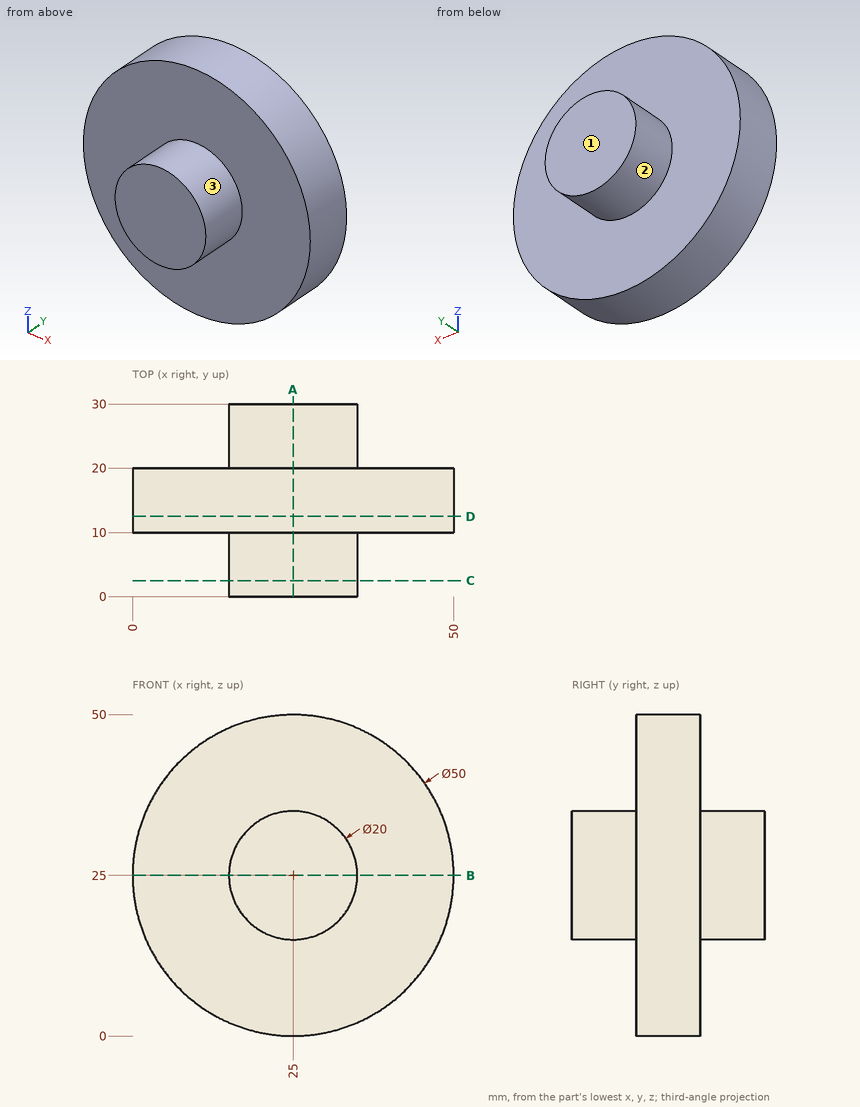
Can you work these out from the drawing? Everything is in mm from the part's minimum corner. A direction names the side the tool comes from. Round coordinates to 2 decimals unless told otherwise and drop trailing zeros. Loops run counter-clockwise (first coordinate to the right, second up) from the corner with the lowest first, then second, coordinate; pieces in that order, holes last. Notation, with made-up numbers: (63.5, 19.25) -> (110.5, 19.25) arc R23 cw to (110.5, 38.25) -> close; hole circle Ø9 at (-6.5, 45). An arc over 180 degrees is marked (long way). Use CSV: the item, a comma, the result in double quotes.
(1) Will these pins go through, and if not, where does the flat tip stop? pin 1 Ø10 at (x, y) = (26, 8.5) entering from +Z; pin 2 Ø6 at (y, z) = (16, 34.5) entering from +X; pin 3 Ø1 at (x, y) = (17.5, 13) entering from -Z.
Return value:
pin 1,"stops at z = 50"
pin 2,"stops at x = 49.14"
pin 3,"stops at z = 1"
(2) Suppose I cut it at C-C on y = 2.5. Write out the boundary of the cut face in (x, z), plus the area to 3 significant figures.
Return value:
outline,"circle Ø20 at (25, 25)"
area,"314 mm²"
(3) For the marked faces 1, 2 and 3, which set-ups out of +Z, -Z, +X, -X, +Y, -Y let a thin tool reach every point of the face, with its end or its side?
Return value:
face 1,"+Z, -Z, +X, -X, +Y"
face 2,"+Y"
face 3,"-Y"
(4) Suppose I cut it at A-A on x = 25. Write out the boundary of the cut face in (y, z), plus the area to 3 significant figures.
Return value:
outline,"(0, 15) -> (10, 15) -> (10, 0) -> (20, 0) -> (20, 15) -> (30, 15) -> (30, 35) -> (20, 35) -> (20, 50) -> (10, 50) -> (10, 35) -> (0, 35) -> close"
area,"900 mm²"
(5) If I drill on probe 1 along Y at (x, z) = (6.5, 14); probe 2 along Z at (x, y) = (22, 13.75); probe 3 along X at (y, z) = (15.75, 33), over which ranges is the centre line in solid material (lowest first)? Write a range as [from, to].
Return value:
probe 1,"y = [10, 20]"
probe 2,"z = [0.18, 49.82]"
probe 3,"x = [1.31, 48.69]"
(6) Suppose I cut it at B-B on z = 25. Write out the boundary of the cut face in (x, y).
Return value:
outline,"(0, 10) -> (15, 10) -> (15, 0) -> (35, 0) -> (35, 10) -> (50, 10) -> (50, 20) -> (35, 20) -> (35, 30) -> (15, 30) -> (15, 20) -> (0, 20) -> close"
(7) Suppose I cut it at D-D on y = 12.5. Write out the boundary of the cut face in (x, z).
Return value:
outline,"circle Ø50 at (25, 25)"
